Could you check a few things on this model? Use its own coordinates, in mm. A direction names the side the tool comes from. Coordinates: 2 decimals unless noted, no trailing zeros. Write each loop counter-clockwise with the first axis right and the second up, starting at its lowest first coordinate (ties: lowest second). Pieces come first, ordered by that corner, then holes.
Autodesk Inventor part; units mm, degrees
ref_plane "YZ Plane" through (0, 0, 0) normal (1, 0, 0) x (0, 1, 0)
ref_plane "XZ Plane" through (0, 0, 0) normal (0, 1, 0) x (-1, 0, 0)
ref_plane "XY Plane" through (0, 0, 0) normal (0, 0, 1) x (1, 0, 0)
sketch "Skizze3" plane through (0, 0, 0) normal (0, 0, 1) x (1, 0, 0)
  line L0 (0, 0) -> (-80, 0)
  line L1 (-80, 0) -> (-80, 100)
  line L2 (-80, 100) -> (0, 100)
  line L3 (0, 100) -> (0, 0)
  line L4 (-80, 100) -> (0, 100)
  line L5 (-40, 105.85) -> (-80, 105.85)
  line L6 (-80, 105.85) -> (-80, 100)
  line L7 (-80, 50) -> (-85.85, 50)
  line L8 (-85.85, 50) -> (-85.85, 98.2)
  line L9 (-85.85, 98.2) -> (-80, 98.2)
  line L10 (-80, 98.2) -> (-80, 50)
  line L11 (-40, 105.85) -> (-40, 100)
  dimension "d4" = 100
  dimension "d5" = 80
  dimension "d6" = 5.85
  dimension "d7" = 5.85
  dimension "d8" = 1.8
extrude "Extrusion3" add sketch "Skizze3" along normal blind 5 contours L0 L1 L2 L3
extrude "Extrusion4" add sketch "Skizze3" along normal blind 5 contours L7 L8 L9 L1 | L2 L6 L5 L11
fillet "Rundung1" radius 2 2 edges at (-85.85, 98.2, 2.5) (-80, 105.85, 2.5)
mirror "Spiegeln1" about plane through (-85.85, 50, 0) normal (0, -1, 0) of "Extrusion4", "Rundung1"
mirror "Spiegeln2" about plane through (-40, 0, 0) normal (1, 0, 0) of "Extrusion4", "Rundung1", "Spiegeln1"
fillet "Rundung2" radius 1.5 4 edges at (-80, 98.2, 2.5) (-80, 1.8, 2.5) (0, 1.8, 2.5) (0, 98.2, 2.5)
equation "\"d7\" = d6"
properties part number "BT701_trajan20_21" material "Acryl"
1. Please list where these lines run through material, in increasing order: line 1 along Y through (x, z) = (-81.5, 0.9); line 2 along X through (y, z) = (2.5, 0.8).
Verdict:
line 1: y = 1.8 to 98.2
line 2: x = -85.37 to 5.37
2. On a 3-axis mill with a long thin cutter (end or side, diameter ignored), from which of +Z, -Z, +X, -X, +Y, -Y can I reach the whole of each face in a straight line? I mean faces 1 (the face through (3, 98.2, 2)), 2 (the face through (-80, -2, 2)), 3 (the face through (3, 1.8, 2)), 4 (the face through (-80, 102, 2)). Say none if no direction works.
Verdict:
face 1: +Z, -Z, +X, +Y
face 2: +Z, -Z, -X, -Y
face 3: +Z, -Z, +X, -Y
face 4: +Z, -Z, -X, +Y
3. I want a section at A-A on z = 2.35. Please give me the cut outline in (x, y), plus the area to 3 significant figures.
Verdict:
outline: (-85.85, 3.8) arc R2 ccw to (-83.85, 1.8) - (-81.5, 1.8) arc R1.5 cw to (-80, 0.3) - (-80, -3.85) arc R2 ccw to (-78, -5.85) - (-2, -5.85) arc R2 ccw to (0, -3.85) - (0, 0.3) arc R1.5 cw to (1.5, 1.8) - (3.85, 1.8) arc R2 ccw to (5.85, 3.8) - (5.85, 96.2) arc R2 ccw to (3.85, 98.2) - (1.5, 98.2) arc R1.5 cw to (0, 99.7) - (0, 103.85) arc R2 ccw to (-2, 105.85) - (-78, 105.85) arc R2 ccw to (-80, 103.85) - (-80, 99.7) arc R1.5 cw to (-81.5, 98.2) - (-83.85, 98.2) arc R2 ccw to (-85.85, 96.2) - close
area: 10,100 mm2
4. For pin 1 (2 mm diameter, centred on y = 101, z = 2.5, fed in from -X); pin 2 (1.9 mm diameter, centred on x = -82.5, z = 2.5, fed in from +Y); pin 3 (2.5 mm diameter, centred on x = 3, z = 3, fed in from -Y), each with a flat end and sliding along its axis, tell me the tip position at first contact or that it passes through.
Verdict:
pin 1: stops at x = -80
pin 2: stops at y = 98.2
pin 3: stops at y = 1.8
